Could you check a few things on this model? Use its own coordinates, in mm. A direction names the side the tool comes from. Coordinates: 2 decimals unless noted, no trailing zeros. Loops run counter-clockwise (first coordinate to the right, second up) from the corner with the lowest first, then second, coordinate; pieces in that order, holes last.
1) Imagine slicing it at B-B on y = -6.5. Please give me the cut outline in (x, z).
2) For faces 1 (the face through (-8.8, -1.6, 45)), 2 (the face through (-4, 0, -46)), 3 (the face through (-50, -7, -48)), which set-ups out of +Z, -Z, +X, -X, +Y, -Y let a thin tool reach every point of the face, with its end or its side?
3) Thinking about a two-plate mould opening in Z: for faces 4 (the face through (-4.1, -12, 50.3)), 5 (the face through (-1, -2, -47)), 6 (the face through (-1, -6, -52)), 7 (the face through (-1, -6, 52)), which applies, released by +Z, released by -Z, zero draft, split by the parting line, or undercut?
4) Imagine slicing it at C-C on z = 31. Please give me the cut outline in (x, y).
5) If I drill on line 1 along Z through (x, y) = (-2, -7.5); line 2 along Z through (x, y) = (5, -1.5); line 3 along X through (y, z) = (-3.5, -27), over which ranges is the centre line in solid material (lowest first)?
6) Will these pins go through, and if not, where does the flat tip stop? P1, Ø5.5, axis at x = -17, z = 47.5, coming from the -Y side; P2, Ø4, axis at x = -21, z = -46.5, coming from the -Y side; P3, Ø4, axis at y = -3, z = -17.5, coming from the -X side.
7) Imagine slicing it at A-A on x = 29.5. Please give me the cut outline in (y, z).
```python
from build123d import *

# Parameters (mm, degrees)
F0_W      = 104
F0_H      = 104
F1_DEPTH  = 2
F2_T      = -2
F3_W      = 104
F3_H      = 2
F4_DEPTH  = 10
F5_W      = 104
F5_H      = 2
F6_DEPTH  = 10
F7_W      = 2
F7_H      = 100
F8_DEPTH  = 10
F9_W      = 2
F9_H      = 100
F10_DEPTH = 10
F13_W     = 111.434492
F13_H     = 90
F14_DEPTH = 25
F15_W     = 15.078314
F15_H     = 90
F16_DEPTH = 25


with BuildPart() as f1:
    # F0 (on Front) → F1 (new body)
    with BuildSketch(Plane.XZ):
        Rectangle(F0_W, F0_H)
    extrude(amount=F1_DEPTH)

    # F2
    f2_openings = [f1.faces().sort_by_distance(p)[0] for p in [
        (0, -2, 0),
    ]]
    offset(amount=F2_T, openings=f2_openings)

    # F3 (on face) → F4 (join)
    with BuildSketch(Plane.XZ.offset(2)):
        with Locations((0, 51)):
            Rectangle(F3_W, F3_H)
    extrude(amount=F4_DEPTH)

    # F5 (on face) → F6 (join)
    with BuildSketch(Plane.XZ.offset(2)):
        with Locations((0, -51)):
            Rectangle(F5_W, F5_H)
    extrude(amount=F6_DEPTH)

    # F7 (on face) → F8 (join)
    with BuildSketch(Plane.XZ.offset(2)):
        with Locations((-51, 0)):
            Rectangle(F7_W, F7_H)
    extrude(amount=F8_DEPTH)

    # F9 (on face) → F10 (join)
    with BuildSketch(Plane.XZ.offset(2)):
        with Locations((51, 0)):
            Rectangle(F9_W, F9_H)
    extrude(amount=F10_DEPTH)

    # F13 (on face) → F14 (cut)
    with BuildSketch(Plane.XZ.offset(2)):
        with Locations((-5.717246, 0)):
            Rectangle(F13_W, F13_H)
    extrude(amount=-F14_DEPTH, mode=Mode.SUBTRACT)

    # F15 (on face) → F16 (cut)
    with BuildSketch(Plane(origin=(-52, 0, 0), x_dir=(0, -1, 0), z_dir=(-1, 0, 0))):
        with Locations((9.539157, 0)):
            Rectangle(F15_W, F15_H)
    extrude(amount=-F16_DEPTH, mode=Mode.SUBTRACT)


solid = f1.part
```
Filled in:
1. outline: (-52, -52) - (52, -52) - (52, 52) - (-52, 52) - (-52, 45) - (-50, 45) - (-50, 50) - (50, 50) - (50, -50) - (-50, -50) - (-50, -45) - (-52, -45) - close
2. face 1: -X, +Y, -Y
2. face 2: +Z, -Z, +X, -X, +Y
2. face 3: -Y
3. face 4: zero draft
3. face 5: undercut
3. face 6: released by -Z
3. face 7: released by +Z
4. outline: (50, -12) - (52, -12) - (52, 0) - (50, 0) - close
5. line 1: z = -52 to -50, 50 to 52
5. line 2: z = -52 to -45, 45 to 52
5. line 3: x = 50 to 52
6. P1: stops at y = -12
6. P2: stops at y = -2
6. P3: stops at x = 50
7. outline: (-12, -52) - (0, -52) - (0, -45) - (-2, -45) - (-2, -50) - (-12, -50) - close; (-12, 50) - (-2, 50) - (-2, 45) - (0, 45) - (0, 52) - (-12, 52) - close
